Can you work these out from the drawing? Everything is in mm from the part's minimum corner. A direction names the side the tool comes from. Round coordinates to 2 decimals unless told otherwise and drop trailing zeros. Loops run counter-clockwise (first coordinate to the right, second up) from the corner with the lowest first, then second, coordinate; pieces in that order, holes last. Notation, with made-up numbers: M -0.75,41 L 50.25,41 A24 ccw 50.25,80 Z; hole C 50,-11 d1. An arc over 180 degrees is marked long. Answer in a Markdown table with one row per item.
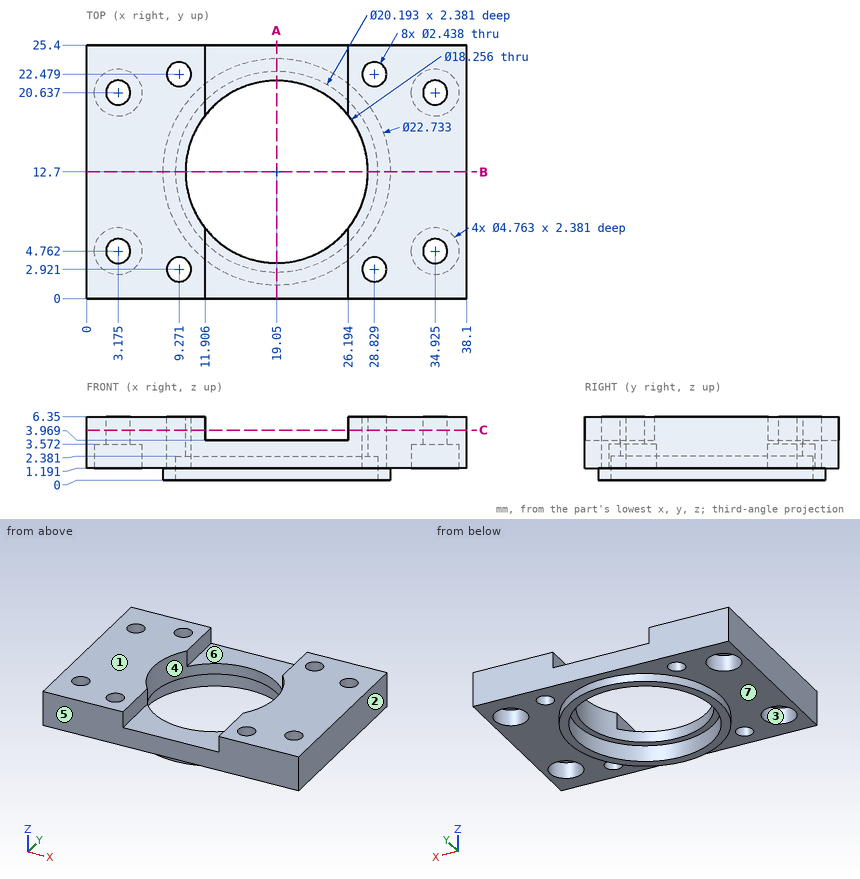
1) I want a section at A-A, the plane x = 19.05. Please give me the cut outline in (y, z).
Computed:
| item | result |
|---|---|
| outline | M 0,1.19 L 1.33,1.19 L 1.33,0 L 2.6,0 L 2.6,2.38 L 3.57,2.38 L 3.57,3.97 L 0,3.97 Z; M 21.83,2.38 L 22.8,2.38 L 22.8,0 L 24.07,0 L 24.07,1.19 L 25.4,1.19 L 25.4,3.97 L 21.83,3.97 Z |
2) Which directions (+Z, -Z, +X, -X, +Y, -Y) give clear straight access to the entire face, cutting with the end or side of a thin tool? Please do the marked faces 5, 6 and 7.
Computed:
| item | result |
|---|---|
| face 5 | +Z, -Z, +X, -X, -Y |
| face 6 | +Z, +Y, -Y |
| face 7 | -Z |
3) I need wall thicknesses on line 1 (X direction, y = 20.5, z = 4.75) (1 decimal); line 2 (X direction, y = 12.7, z = 4.7); line 3 (X direction, y = 6.25, z = 4.75). Which ranges of each line are inside material? Lowest first, please.
Computed:
| item | result |
|---|---|
| line 1 | x = 0 to 2, 4.4 to 11.9, 26.2 to 33.7, 36.1 to 38.1 |
| line 2 | x = 0 to 9.92, 28.18 to 38.1 |
| line 3 | x = 0 to 11.91, 26.19 to 38.1 |
4) I want a section at C-C, the plane z = 5. State how many separate pieces and enclosed holes the cut face has.
Computed:
| item | result |
|---|---|
| separate pieces | 2 |
| enclosed holes | 8 |
5) If we mould it in two halves opening along X, with no side actions, what happens to the marked faces 1, 2, 3 and 4? For each: released by +X, released by -X, zero draft, split by the parting line, or undercut.
Computed:
| item | result |
|---|---|
| face 1 | zero draft |
| face 2 | released by +X |
| face 3 | undercut |
| face 4 | undercut |
6) Will these pins go through, and if not, where does the flat tip stop? P1, Ø5.5, axis at x = 19, y = 3.5, coming from the +Z side; P2, Ø5, axis at x = 35.5, y = 3.5, coming from the -Z side; P3, Ø4.5, axis at x = 34.92, y = 4.76, coming from the -Z side.
Computed:
| item | result |
|---|---|
| P1 | stops at z = 3.97 |
| P2 | stops at z = 1.19 |
| P3 | stops at z = 3.57 |
7) I want a section at B-B, the plane y = 12.7. Please give me the cut outline in (x, z), plus the area to 3 significant figures.
Computed:
| item | result |
|---|---|
| outline | M 0,1.19 L 7.68,1.19 L 7.68,0 L 8.95,0 L 8.95,2.38 L 9.92,2.38 L 9.92,6.35 L 0,6.35 Z; M 28.18,2.38 L 29.15,2.38 L 29.15,0 L 30.42,0 L 30.42,1.19 L 38.1,1.19 L 38.1,6.35 L 28.18,6.35 Z |
| area | 103 mm² |
